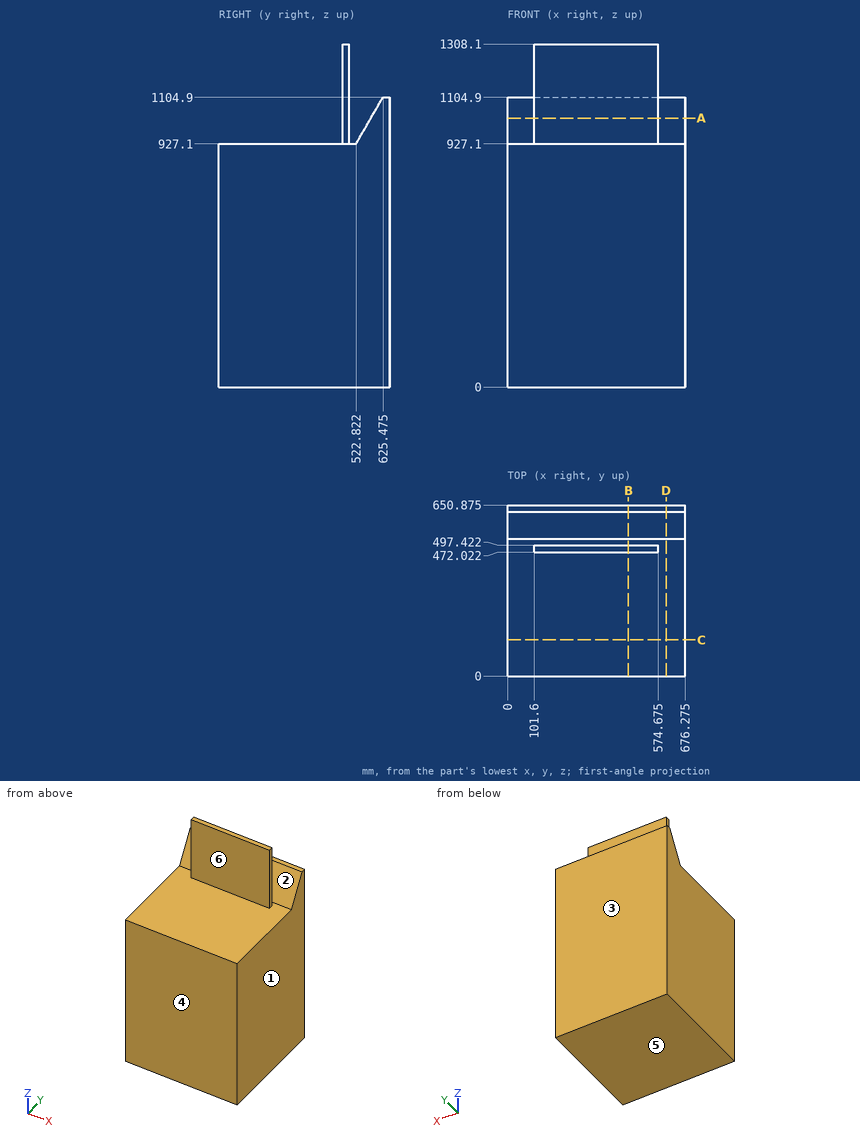
Geometry check sheet. Reference: drawing and pictorial views, mm from the part's lowest x, y, z. A direction names the side the tool comes from. Coordinates: 2 decimals unless noted, no trailing zeros. Loops run counter-clockwise (first coordinate to the right, second up) from the corner with the lowest first, then second, coordinate; pieces in that order, holes last.
1) Sectioned sample at A-A (z = 1026). Record the boundary of the cut face in (x, y) (3 decimals).
2) Access from +Z, -Z, +X, -X, +Y, -Y to the whole of each face (thin tool, end or side, straight path). Record for the marked faces 5 and 6.
3) Material ranges on probe 1 along Y at (x, z) = (151, 1016.5) (1 decimal); probe 2 along Z at (x, y) = (534, 95.5); probe 3 along Y at (x, z) = (189.5, 1102.5) (1 decimal), recorded low to high.
4) Release check for a two-part mould opening along Y. For the marked faces 1, 2, 3 and 4 record: released by +Y, released by -Y, zero draft, split by the parting line, or undercut.
5) Sectioned sample at B-B (x = 460.5). Record the boundary of the cut face in (y, z) (3 decimals), and give its area (3 significant figures).
6) Gauge pin test, flat ends, axial feed: pin 1 (12.5 mm diameter, centred on y = 488, z = 1035, fed in from -X); pin 2 (6 mm diameter, centred on x = 177, y = 252.5, fed in from +Z); pin 3 (7.5 mm diameter, centred on x = 450, y = 644.5, fed in from +Z). Record the tip position at first contact, or that the pin passes through.
7) Sectioned sample at C-C (y = 138). Record the boundary of the cut face in (x, z) (3 decimals), and give its area (3 significant figures).
8) Sectioned sample at D-D (x = 604). Record the boundary of the cut face in (y, z) (3 decimals), and give its area (3 significant figures).
Check sheet entries:
1. outline: (0, 579.922) - (676.275, 579.922) - (676.275, 650.875) - (0, 650.875) - close; (101.6, 472.022) - (574.675, 472.022) - (574.675, 497.422) - (101.6, 497.422) - close
2. face 5: -Z, +X, -X, +Y, -Y
2. face 6: +Z, +X, -X, -Y
3. probe 1: y = 472 to 497.4, 574.4 to 650.9
3. probe 2: z = 0 to 927.1
3. probe 3: y = 472 to 497.4, 624.1 to 650.9
4. face 1: zero draft
4. face 2: undercut
4. face 3: released by +Y
4. face 4: released by -Y
5. outline: (0, 0) - (650.875, 0) - (650.875, 1104.9) - (625.475, 1104.9) - (522.822, 927.1) - (497.422, 927.1) - (497.422, 1308.1) - (472.022, 1308.1) - (472.022, 927.1) - (0, 927.1) - close
5. area: 627,000 mm2
6. pin 1: stops at x = 101.6
6. pin 2: stops at z = 927.1
6. pin 3: stops at z = 1104.9
7. outline: (0, 0) - (676.275, 0) - (676.275, 927.1) - (0, 927.1) - close
7. area: 627,000 mm2
8. outline: (0, 0) - (650.875, 0) - (650.875, 1104.9) - (625.475, 1104.9) - (522.822, 927.1) - (0, 927.1) - close
8. area: 617,000 mm2
